The figure shows three views and two pictorial views of one solid part (mm, origin at its lowest corner). Answer the questions. A direction names the side the tool comes from. Coordinates: 2 decimals unless noted, no trailing zeros. Loops run counter-clockwise (first coordinate to the right, second up) from the corner with the lowest first, then second, coordinate; pieces in that order, holes last. Notation, with made-up numbers: (49.25, 46.5) -> (70.25, 46.5) arc R23 ccw to (70.25, 73.5) -> close; hole circle Ø7 at (-20, -31.5). An arc over 180 degrees is marked (long way). Answer in a Markdown table with one row per item.
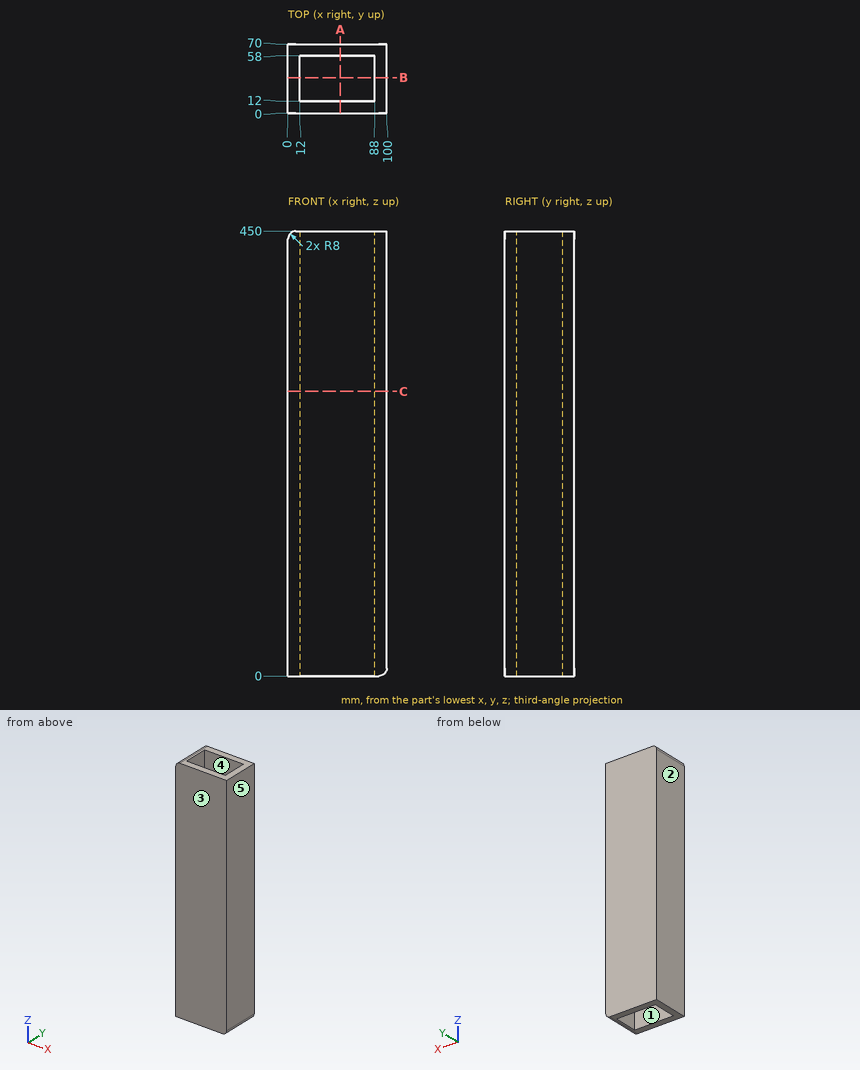
Item 1: Determine the mould class of the marked faces 1, 2 and 3 for opening direction X: +X half, -X half, draft (parallel to the pull), parting line (faces both ways), or undercut.
Findings below:
| item | result |
|---|---|
| face 1 | undercut |
| face 2 | -X half |
| face 3 | draft |
Item 2: A tool of negligible diameter and unlimited length cuts with its end or side. For the marked faces 4 and 5, from which of +Z, -Z, +X, -X, +Y, -Y can it reach the whole face along a straight path? Write none if from no direction.
Findings below:
| item | result |
|---|---|
| face 4 | +Z, -Z |
| face 5 | +Z, -Z, +X, +Y, -Y |
Item 3: A cutting plane is placed at B-B, the plane y = 36. Determine the outline of the cut face in (x, z).
Findings below:
| item | result |
|---|---|
| outline | (0, 0) -> (12, 0) -> (12, 450) -> (8, 450) arc R8 ccw to (0, 442) -> close; (88, 0) -> (92, 0) arc R8 ccw to (100, 8) -> (100, 450) -> (88, 450) -> close |
Item 4: A cutting plane is placed at C-C, the plane z = 288. Determine the outline of the cut face in (x, y), plus the area to 3 significant figures.
Findings below:
| item | result |
|---|---|
| outline | (0, 0) -> (100, 0) -> (100, 70) -> (0, 70) -> close; hole (12, 12) -> (88, 12) -> (88, 58) -> (12, 58) -> close |
| area | 3,500 mm2 |
Item 5: Find the intervals of material crossed by probe 1 along X at (y, z) = (42.5, 222); probe 2 along Y at (x, z) = (40, 231); probe 3 along Z at (x, y) = (94.5, 22.5), in increasing order.
Findings below:
| item | result |
|---|---|
| probe 1 | x = 0 to 12, 88 to 100 |
| probe 2 | y = 0 to 12, 58 to 70 |
| probe 3 | z = 0.4 to 450 |
Item 6: A cutting plane is placed at A-A, the plane x = 53. Determine the outline of the cut face in (y, z).
Findings below:
| item | result |
|---|---|
| outline | (0, 0) -> (12, 0) -> (12, 450) -> (0, 450) -> close; (58, 0) -> (70, 0) -> (70, 450) -> (58, 450) -> close |
Item 7: A flat-ended cylindrical pin translates along its axis: pin 1 Ø1 at (x, z) = (54, 389) entering from -Y. Find the tip coordinate at first contact, or state that the pin passes through.
Findings below:
| item | result |
|---|---|
| pin 1 | stops at y = 0 |
